Part model, mm, in its own coordinate system. Give positions to 0.01 mm unless a question says otherwise; leave off trailing zeros. Loops run counter-clockwise (first coordinate to the right, second up) from the corner with the lowest first, then second, coordinate; pieces in that order, holes last. Notation, with made-up numbers: (-39, -33.75) -> (-30, -33.75) arc R23 ccw to (-30, -12.75) -> close; hole circle Ø3 at (55.25, 71.5). An arc over 180 degrees is marked (long way). Write item = value, one per line.
Autodesk Inventor part; units mm, degrees
ref_plane "YZ Plane" through (0, 0, 0) normal (1, 0, 0) x (0, 1, 0)
ref_plane "XZ Plane" through (0, 0, 0) normal (0, 1, 0) x (-1, 0, 0)
ref_plane "XY Plane" through (0, 0, 0) normal (0, 0, 1) x (1, 0, 0)
sketch "Sketch2" plane through (0, 0, 0) normal (0, 1, 0) x (-1, 0, 0)
  line L0 (48.5, 48.5) -> (-48.5, 48.5)
  line L1 (-48.5, 48.5) -> (-48.5, -48.5)
  line L2 (-48.5, -48.5) -> (48.5, -48.5)
  line L3 (48.5, -48.5) -> (48.5, 48.5)
  circle A0 centre (0, 27) radius 22
  line L4 (48.5, -48.5) -> (18.25, -48.5)
  line L5 (18.25, -48.5) -> (18.25, 6.5)
  line L6 (18.25, 6.5) -> (48.5, 6.5)
  line L7 (48.5, 6.5) -> (48.5, -48.5)
  line L8 (-48.5, -48.5) -> (-18.25, -48.5)
  line L9 (-18.25, -48.5) -> (-18.25, 6.5)
  line L10 (-18.25, 6.5) -> (-48.5, 6.5)
  line L11 (-48.5, 6.5) -> (-48.5, -48.5)
  line L12 (21.25, 6.5) -> (18.25, 3.5)
  line L13 (-18.25, 3.5) -> (-21.25, 6.5)
  point P0 (0, 0)
  point P1 (-48.5, 6.5)
  point P2 (18.25, -48.5)
  point P3 (48.5, 6.5)
  dimension "d1" = 44
  dimension "d2" = 97
  dimension "d3" = 97
  dimension "d4" = 48.5
  dimension "d5" = 48.5
  dimension "d8" = 30.25
  dimension "d9" = 30.25
  dimension "d10" = 55
  dimension "d11" = 55
  dimension "d14" = 0
  dimension "d15" = 45
  dimension "d16" = 3
  dimension "d17" = 3
  dimension "d18" = 21.5
  dimension "d19" = 27
extrude "Extrusion1" add sketch "Sketch2" along normal blind 1.6 contours L3 L6 L5 L2 L9 L10 L1 L0 A0 | L12 L5 L6 | L10 L9 L13
properties part number "pcb" material "UHMW, Black"
1) Drop flat-ended pins along their axis: P1, Ø0.8, axis at x = 36, y = 1, coming from the -Z side; P2, Ø0.8, axis at y = 1, z = -21.5, coming from the +X side; P3, Ø0.5, axis at y = 0.5, z = -17, coming from the -X side. Give the stop position or say it passes through.
Resolved:
P1 = 6.5
P2 = 18.25
P3 = -18.25
2) Slice it at D-D, the plane x = -32.5. List the corners of the cut face in (y, z), and give its area (3 significant figures).
Resolved:
outline = (0, 6.5) -> (1.6, 6.5) -> (1.6, 48.5) -> (0, 48.5) -> close
area = 67.2 mm²
3) Slice it at A-A, the plane z = 27. List the corners of the cut face in (x, y).
Resolved:
outline = (-48.5, 0) -> (-22, 0) -> (-22, 1.6) -> (-48.5, 1.6) -> close; (22, 0) -> (48.5, 0) -> (48.5, 1.6) -> (22, 1.6) -> close
4) Slice it at C-C, the plane x = 12. List the corners of the cut face in (y, z).
Resolved:
outline = (0, -48.5) -> (1.6, -48.5) -> (1.6, 8.56) -> (0, 8.56) -> close; (0, 45.44) -> (1.6, 45.44) -> (1.6, 48.5) -> (0, 48.5) -> close
5) Slice it at B-B, the plane y = 0.85. List the corners of the cut face in (x, z).
Resolved:
outline = (-48.5, 6.5) -> (-21.25, 6.5) -> (-18.25, 3.5) -> (-18.25, -48.5) -> (18.25, -48.5) -> (18.25, 3.5) -> (21.25, 6.5) -> (48.5, 6.5) -> (48.5, 48.5) -> (4.66, 48.5) arc R22 cw (long way) to (-4.66, 48.5) -> (-48.5, 48.5) -> close
6) Pull direction X, two halves, no side cores. Call faces 1 (the face through (-0.9, 0.79, 5.02)), 2 (the face through (1, 1.6, 1)), 3 (the face through (19.73, 0.79, 4.98)): pulls with the +X half, pulls with the -X half, needs draft (parallel to the pull), parting line crosses it, or undercut.
Resolved:
face_1 = undercut
face_2 = needs draft
face_3 = pulls with the +X half
7) Drill centre lines: line 1 along X through (y, z) = (1.25, 27); line 2 along X through (y, z) = (1.5, -27); line 3 along Z through (x, y) = (0, 0.7). Where is each one in solid material? Low to high. Write a range as [from, to].
Resolved:
line_1 = [-48.5, -22], [22, 48.5]
line_2 = [-18.25, 18.25]
line_3 = [-48.5, 5]
